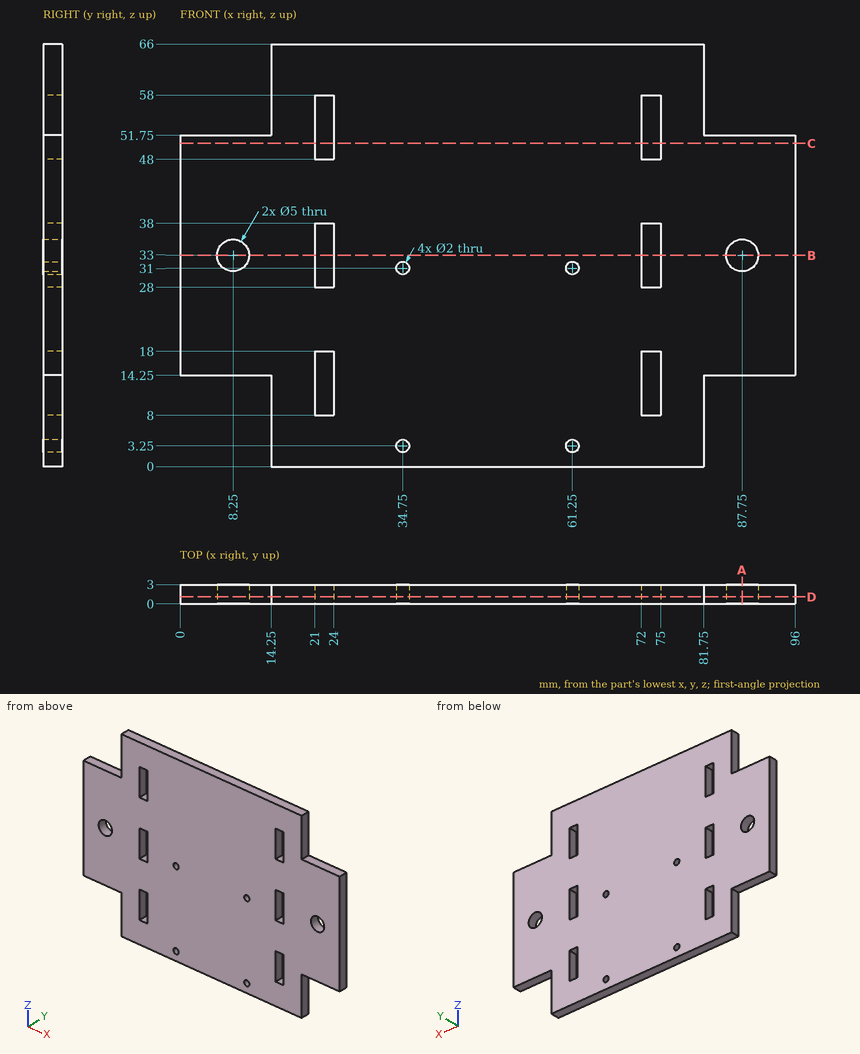
Study the drawing (mm; zero at the part's minimum x, y, z) and answer. Round coordinates to 2 decimals unless told otherwise and drop trailing zeros. Order: outer loops, then holes, each group sorted by start corner. A loop starts at its lowest first (then second) coordinate and runs counter-clockwise, first axis right, second up. Notation, with made-up numbers: (48, 49) - (59, 49) arc R16 cw to (59, 69) - close; hole circle Ø10 at (4, -22). An arc over 180 degrees is marked (long way). Use one line per item in the form item = value. Start each with the question number.
(1) The part is cut by section C-C (z = 50.5). Give the vertices of the cut face in (x, y).
(2) The part is cut by section A-A (x = 87.75). Give the vertices of the cut face in (y, z).
(3) Find the intervals of material crossed by line 1 along X through (y, z) = (0.85, 11); line 2 along X through (y, z) = (0.9, 33); line 3 along X through (y, z) = (2.1, 3.25), in increasing order. Write a range as from..to.
(4) The part is cut by section B-B (z = 33). Give the vertices of the cut face in (x, y).
(5) Flat-ended cylindrical pins translate along their axes: pin 1 Ø6 at (x, z) = (84, 41) entering from -Y; pin 2 Ø1.5 at (x, y) = (11.5, 1) entering from -Z. Find the tip coordinate at first contact, or state that the pin passes through.
(6) The part is cut by section D-D (y = 1.1). Count the separate pieces of the cut face and the enclosed holes in it, then the cut area to 3 significant figures.
Checked values:
q1.outline = (0, 0) - (21, 0) - (21, 3) - (0, 3) - close; (24, 0) - (72, 0) - (72, 3) - (24, 3) - close; (75, 0) - (96, 0) - (96, 3) - (75, 3) - close
q2.outline = (0, 14.25) - (3, 14.25) - (3, 30.5) - (0, 30.5) - close; (0, 35.5) - (3, 35.5) - (3, 51.75) - (0, 51.75) - close
q3.line_1 = 14.25..21, 24..72, 75..81.75
q3.line_2 = 0..5.75, 10.75..21, 24..72, 75..85.25, 90.25..96
q3.line_3 = 14.25..33.75, 35.75..60.25, 62.25..81.75
q4.outline = (0, 0) - (5.75, 0) - (5.75, 3) - (0, 3) - close; (10.75, 0) - (21, 0) - (21, 3) - (10.75, 3) - close; (24, 0) - (72, 0) - (72, 3) - (24, 3) - close; (75, 0) - (85.25, 0) - (85.25, 3) - (75, 3) - close; (90.25, 0) - (96, 0) - (96, 3) - (90.25, 3) - close
q5.pin_1 = 0
q5.pin_2 = 14.25
q6.separate_pieces = 1
q6.enclosed_holes = 12
q6.area = 5,290 mm^2
